Part model, mm, in its own coordinate system. A direction names the side the tool comes from. Give positions to 0.01 mm unless a question says otherwise; leave off trailing zeros. Order: outer loops, then holes, each group sorted by start corner. A loop starts at its lowest first (then second) coordinate and runs counter-clockwise, first axis right, second up.
1. Slice it at A-A on y = 3.5. List the corners of the cut face in (x, z), and give its area (3 significant figures).
2. Drop flat-ended pins along their axis: pin 1 Ø3 at (y, z) = (35, 24.5) entering from -X; pin 2 Ø5 at (y, z) = (7, 3.5) entering from +X; pin 3 Ø4 at (y, z) = (24, 5) entering from -X; pin 4 Ø0.9 at (x, z) = (2, 9) entering from +Y. Give the stop position or say it passes through.
3. Which spindle directions (+Z, -Z, +X, -X, +Y, -Y) get a long thin tool onto all of the face, cutting with end or side? Do faces 1 (the cylindrical face through (7, 5.4, 23.3)), 2 (the flat face through (4.5, 20, 14)), 3 (the flat face through (1, 21, 14)). Say none if no direction does.
4. Probe line 1 (Z direction, x = 8.05, y = 7); line 2 (X direction, y = 11, z = 7.25); line 3 (X direction, y = 6, z = 4.75). List the from-to ranges inside material, lowest first.
5. Slice it at D-D on y = 35. List the corners of the cut face in (x, z).
6. Mould opens along Z. For faces 4 (the flat face through (5, 0, 14)), 5 (the cylindrical face through (7.035, 36.847, 23.734)), 6 (the cylindrical face through (4.684, 0.285, 27.699)) say: +Z half, -Z half, draft (parallel to the pull), parting line (faces both ways), or undercut.
7. Slice it at C-C on z = 3.5. List the corners of the cut face in (x, y), and give its area (3 significant figures).
8. Slice it at B-B on x = 7.75. List the corners of the cut face in (y, z), and give its area (3 significant figures).
from build123d import *

# Parameters (mm, degrees)
PAD_DEPTH    = 28
SKETCH001_R  = 2
POCKET_DEPTH = 5
FILLET_R     = 1


with BuildPart() as part:
    # Sketch → Pad (new body)
    with BuildSketch(Plane.XY):
        Polygon((0, 0), (0, 21), (3, 21), (3, 3), (4.5, 3), (4.5, 38), (9.5, 38), (9.5, 0), align=None)
    extrude(amount=PAD_DEPTH)

    # Sketch001 (on Face7 of Pad) → Pocket (cut)
    with BuildSketch(Plane.YZ.offset(9.5)):
        with Locations((7, 24.5)):
            Circle(SKETCH001_R)
        with Locations((35, 24.5)):
            Circle(SKETCH001_R)
        with Locations((7, 3.5)):
            Circle(SKETCH001_R)
        with Locations((35, 3.5)):
            Circle(SKETCH001_R)
    extrude(amount=-POCKET_DEPTH, mode=Mode.SUBTRACT)

    # Fillet
    fillet_edges = [part.edges().sort_by_distance(p)[0] for p in [
        (9.5, 0, 14),
        (0, 0, 14),
        (4.75, 0, 0),
        (4.75, 0, 28),
    ]]
    fillet(fillet_edges, radius=FILLET_R)


solid = part.part
Data:
1. outline: (0, 0) - (3, 0) - (3, 28) - (0, 28) - close; (4.5, 0) - (9.5, 0) - (9.5, 28) - (4.5, 28) - close
1. area: 224 mm2
2. pin 1: passes through
2. pin 2: stops at x = 9.5
2. pin 3: stops at x = 4.5
2. pin 4: stops at y = 21
3. face 1: +X
3. face 2: +Z, -Z, +Y
3. face 3: +Z, -Z, -X, +Y
4. line 1: z = 0 to 1.5, 5.5 to 22.5, 26.5 to 28
4. line 2: x = 0 to 3, 4.5 to 9.5
4. line 3: x = 0 to 3
5. outline: (4.5, 0) - (9.5, 0) - (9.5, 1.5) - (4.5, 1.5) - close; (4.5, 5.5) - (9.5, 5.5) - (9.5, 22.5) - (4.5, 22.5) - close; (4.5, 26.5) - (9.5, 26.5) - (9.5, 28) - (4.5, 28) - close
6. face 4: draft
6. face 5: undercut
6. face 6: +Z half
7. outline: (0, 1) arc R1 ccw to (1, 0) - (8.5, 0) arc R1 ccw to (9.5, 1) - (9.5, 5) - (4.5, 5) - (4.5, 3) - (3, 3) - (3, 21) - (0, 21) - close; (4.5, 9) - (9.5, 9) - (9.5, 33) - (4.5, 33) - close; (4.5, 37) - (9.5, 37) - (9.5, 38) - (4.5, 38) - close
7. area: 217 mm2
8. outline: (0, 1) arc R1 ccw to (1, 0) - (38, 0) - (38, 28) - (1, 28) arc R1 ccw to (0, 27) - close; hole circle Ø4 at (7, 3.5); hole circle Ø4 at (7, 24.5); hole circle Ø4 at (35, 3.5); hole circle Ø4 at (35, 24.5)
8. area: 1,010 mm2
